The model under review builds one solid part; all positions refer to its coordinate system, in mm. A direction names the side the tool comes from. Give positions to 0.01 mm unless a question says otherwise; leave off trailing zeros. Order: outer loops, then holes, each group sorted by start corner. A loop starts at its lowest first (then second) coordinate and runs counter-clockwise, first axis right, second up. Notation, with made-up numbers: (-5.5, 71) -> (30.5, 71) arc R17 cw to (30.5, 104) -> close; hole circle Ø10 at (-9.5, 37). An arc over 180 degrees is marked (long way). Use one line per item in the form item = value.
```python
from build123d import *

# Parameters (mm, degrees)
F0_R     = 4.7371
F1_DEPTH = 7.9502
F2_R     = 6.35
F3_R     = 3.175


with BuildPart() as f1:
    # F0 (on Front) → F1 (new body)
    with BuildSketch(Plane.XZ):
        with BuildLine():
            Line((-7.9375, 0), (-22.1234, 0))
            ThreePointArc((-22.1234, 0), (0, -22.1234), (22.1234, 0))
            Line((22.1234, 0), (7.9375, 0))
            Line((7.9375, 0), (7.9375, 20.650446))
            ThreePointArc((7.9375, 20.650446), (0, 22.1234), (-7.9375, 20.650446))
            Line((-7.9375, 20.650446), (-7.9375, 0))
        make_face()
        Circle(F0_R, mode=Mode.SUBTRACT)
        with BuildLine():
            ThreePointArc((-4.747236, 14.3002), (0, 19.4437), (4.747236, 14.3002))
            ThreePointArc((4.747236, 14.3002), (0, 9.1567), (-4.747236, 14.3002))
        make_face(mode=Mode.SUBTRACT)
    extrude(amount=F1_DEPTH)

    # F2
    f2_edges = [f1.edges().sort_by_distance(p)[0] for p in [
        (-7.9375, -3.9751, 0),
        (7.9375, -3.9751, 0),
    ]]
    fillet(f2_edges, radius=F2_R)

    # F3
    f3_edges = [f1.edges().sort_by_distance(p)[0] for p in [
        (22.1234, -3.9751, 0),
        (-22.1234, -3.9751, 0),
    ]]
    fillet(f3_edges, radius=F3_R)


solid = f1.part
```
1. Add section B-B on y = -1. Count the separate pieces of the cut face and the enclosed holes in it, then the cut area to 3 significant figures.
Values:
separate_pieces = 1
enclosed_holes = 2
area = 975 mm^2
2. Add section A-A on x = 0. Give the boundary of the cut face in (y, z), then the cut area to 3 significant figures.
Values:
outline = (-7.95, -22.12) -> (0, -22.12) -> (0, -4.74) -> (-7.95, -4.74) -> close; (-7.95, 4.74) -> (0, 4.74) -> (0, 9.16) -> (-7.95, 9.16) -> close; (-7.95, 19.44) -> (0, 19.44) -> (0, 22.12) -> (-7.95, 22.12) -> close
area = 195 mm^2
3. For pin 1 Ø3.5 at (x, y) = (-16.5, -5) entering from +Z; pin 2 Ø2 at (x, y) = (-17.5, -6.5) entering from -Z; pin 3 Ø1 at (x, y) = (1.5, -3.5) entering from -Z, all flat-tipped, find the tip position at first contact; note any pin that passes through.
Values:
pin_1 = 0
pin_2 = -14.74
pin_3 = -22.1
4. The part is to be moulded in two halves that separate along X. For faces 5 (the face through (0.114, -3.919, 22.123)), 6 (the face through (21.131, -4.031, -1.156)), 7 (the face through (-21.081, -4.031, -1.097)), 8 (the face through (0.11, -3.919, 9.158)), say which applies: +X half, -X half, draft (parallel to the pull), parting line (faces both ways), or undercut.
Values:
face_5 = parting line
face_6 = +X half
face_7 = -X half
face_8 = undercut
5. Tool access review of faces 1 (the face through (17, -4, 0)), 2 (the face through (-7.938, -4, 14)), 3 (the face through (0, 0, -10)), 4 (the face through (-0.11, -3.919, 19.442)): name each direction out of +Z, -Z, +X, -X, +Y, -Y from which nothing blocks a thin tool from reaching the whole face with its end or side.
Values:
face_1 = +Z, +X, +Y, -Y
face_2 = +Z, -X, +Y, -Y
face_3 = +Z, -Z, +X, -X, +Y
face_4 = +Y, -Y
6. Add section C-C on z = 4. Give the boundary of the cut face in (x, y).
Values:
outline = (-8.39, -7.95) -> (-2.54, -7.95) -> (-2.54, 0) -> (-8.39, 0) -> close; (2.54, -7.95) -> (8.39, -7.95) -> (8.39, 0) -> (2.54, 0) -> close
7. For L1, parallel to X at y = -7.5, z = -2.5; L2, parallel to X at y = -6.5, z = 13; L3, parallel to X at y = -2.5, z = 8, list the stretches that pass through material, from the lowest coordinate up.
Values:
L1 = -21.78 to -4.02, 4.02 to 21.78
L2 = -7.94 to -4.67, 4.67 to 7.94
L3 = -7.94 to 7.94
8. Add section D-D on z = 10. Give the boundary of the cut face in (x, y), then the cut area to 3 significant figures.
Values:
outline = (-7.94, -7.95) -> (-2.71, -7.95) -> (-2.71, 0) -> (-7.94, 0) -> close; (2.71, -7.95) -> (7.94, -7.95) -> (7.94, 0) -> (2.71, 0) -> close
area = 83.2 mm^2
